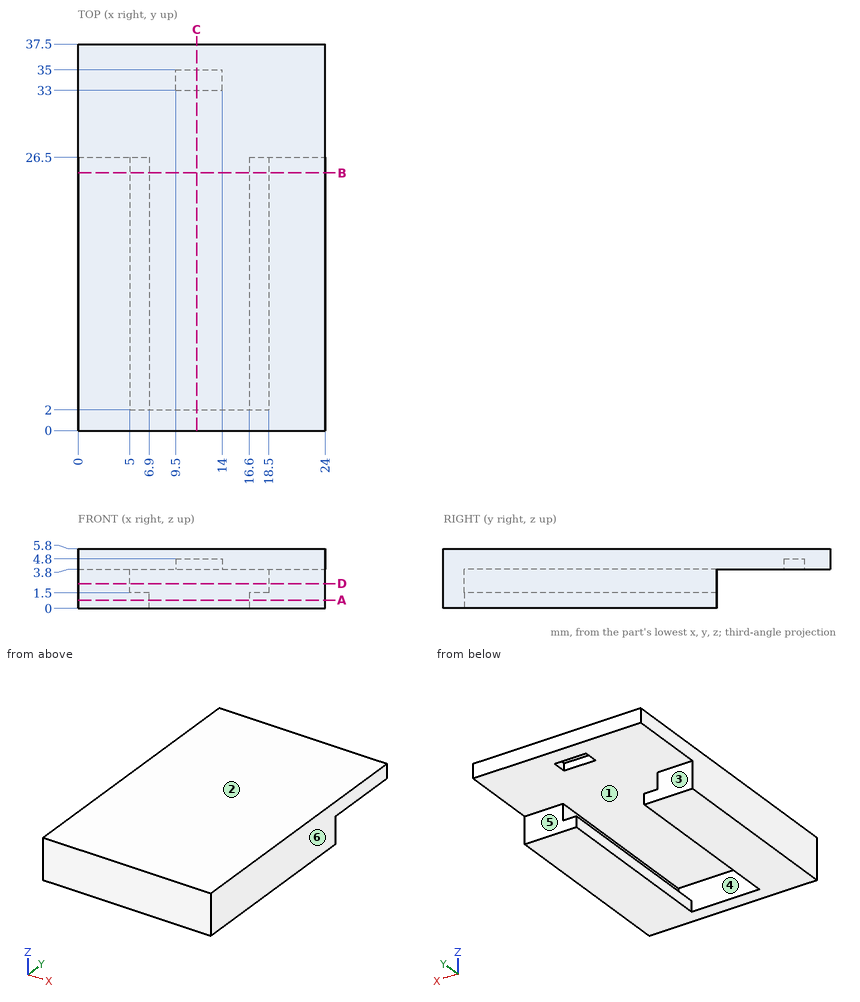
Verification items for this drawing (mm, ordinates from the low corner). A direction names the side the tool comes from. Coordinates: 2 decimals unless noted, no trailing zeros. Write each loop counter-clockwise with the first axis right and the second up, starting at its lowest first coordinate (ties: lowest second). Pieces come first, ordered by that corner, then holes. Notation, with made-up numbers: M 50,72 L 56,72 A14 cw 56,92 Z; hole C 63.25,-37.5 d1. An arc over 180 degrees is marked long. Answer as CSV lines item,"result".
Q1. Cross-section at A-A (z = 0.8). Record the boundary of the cut face in (x, y).
Check result:
outline,"M 0,0 L 24,0 L 24,26.5 L 16.6,26.5 L 16.6,2 L 6.9,2 L 6.9,26.5 L 0,26.5 Z"
Q2. Set-up check for the marked faces 1, 2 and 3: record each of +Z, -Z, +X, -X, +Y, -Y from which the full face is reachable in a straight line by a thin tool's end or side.
Check result:
face 1,"+Y"
face 2,"+Z, +X, -X, +Y, -Y"
face 3,"-Z, +X, -X, +Y"
Q3. Mould release check, pull along X, two halves, no side actions. Record for the marked faces 4, 5 and 6: released by +X, released by -X, zero draft, split by the parting line, or undercut.
Check result:
face 4,"undercut"
face 5,"zero draft"
face 6,"released by +X"
Q4. Go/stop test with flat-tipped pins: pin 1 (2 mm diameter, centred on x = 12.5, y = 13.5, fed in from -Z); pin 2 (3 mm diameter, centred on x = 2, z = 1, fed in from +Y). Record where each tip stops, or that it passes through.
Check result:
pin 1,"z = 3.8"
pin 2,"y = 26.5"
Q5. Cross-section at B-B (y = 25). Record the boundary of the cut face in (x, z), then the cut area to 3 significant figures.
Check result:
outline,"M 0,0 L 6.9,0 L 6.9,1.5 L 5,1.5 L 5,3.8 L 18.5,3.8 L 18.5,1.5 L 16.6,1.5 L 16.6,0 L 24,0 L 24,5.8 L 0,5.8 Z"
area,"93.6 mm^2"
Q6. Material ranges on probe 1 along X at (y, z) = (10, 1.55); probe 2 along X at (y, z) = (5, 1.35); probe 3 along Z at (x, y) = (6.25, 16), recorded low to high. Write a range as from..to.
Check result:
probe 1,"0..5, 18.5..24"
probe 2,"0..6.9, 16.6..24"
probe 3,"0..1.5, 3.8..5.8"
Q7. Cross-section at D-D (z = 2.4). Record the boundary of the cut face in (x, y), then the cut area to 3 significant figures.
Check result:
outline,"M 0,0 L 24,0 L 24,26.5 L 18.5,26.5 L 18.5,2 L 5,2 L 5,26.5 L 0,26.5 Z"
area,"305 mm^2"
Q8. Cross-section at C-C (x = 11.5). Record the boundary of the cut face in (y, z), then the cut area to 3 significant figures.
Check result:
outline,"M 0,0 L 2,0 L 2,3.8 L 33,3.8 L 33,4.8 L 35,4.8 L 35,3.8 L 37.5,3.8 L 37.5,5.8 L 0,5.8 Z"
area,"80.6 mm^2"
